```python
from build123d import *

# Parameters (mm, degrees)
SKETCH1_W               = 15
SKETCH1_H               = 7.5
BOSS_EXTRUDE_BASE_DEPTH = 3
SKETCH2_W               = 15
SKETCH2_H               = 2.5
SKETCH2_H_2             = 1.4
BOSS_EXTRUDE2_DEPTH     = 16
CUT_EXTRUDE1_DEPTH      = 26.342651795
SKETCH6_R               = 2.75
CUT_EXTRUDE_HOLE_DEPTH  = 26.342651795
SKETCH7_R               = 5.5
BOSS_EXTRUDE4_DEPTH     = 3
CUT_EXTRUDE4_DEPTH      = 3


with BuildPart() as part:
    # Sketch1 → Boss-Extrude - Base (new body)
    with BuildSketch(Plane(origin=(0, 0, 0), x_dir=(1, 0, 0), z_dir=(0, 1, 0))):
        with Locations((7.5, 3.75)):
            Rectangle(SKETCH1_W, SKETCH1_H)
    extrude(amount=BOSS_EXTRUDE_BASE_DEPTH)

    # Sketch2 → Boss-Extrude2 (add)
    with BuildSketch(Plane(origin=(0, 3, 0), x_dir=(1, 0, 0), z_dir=(0, 1, 0))):
        with Locations((7.5, 6.25)):
            Rectangle(SKETCH2_W, SKETCH2_H)
        with Locations((7.5, 0.7)):
            Rectangle(SKETCH2_W, SKETCH2_H_2)
    extrude(amount=BOSS_EXTRUDE2_DEPTH)

    # Sketch4 → Cut-Extrude1 (cut, through all)
    with BuildSketch(Plane(origin=(0, 0, -7.5), x_dir=(-1, 0, 0), z_dir=(0, 0, -1))):
        with BuildLine():
            Line((0, 3), (3.144969959, 3))
            Line((3.144969959, 3), (3.144969959, 20.655431795))
            Line((3.144969959, 20.655431795), (-18.154935256, 20.655431795))
            Line((-18.154935256, 20.655431795), (-18.154935256, 3))
            Line((-18.154935256, 3), (-15, 3))
            ThreePointArc((-15, 3), (-14.902566102, 3.529038543), (-14.623050239, 3.988653628))
            ThreePointArc((-14.623050239, 3.988653628), (-13.75, 5.91762732), (-14.133249581, 8))
            ThreePointArc((-14.133249581, 8), (-7.5, 19), (-0.866750419, 8))
            ThreePointArc((-0.866750419, 8), (-1.25, 5.91762732), (-0.376949761, 3.988653628))
            ThreePointArc((-0.376949761, 3.988653628), (-0.097433898, 3.529038543), (0, 3))
        make_face()
    extrude(amount=-CUT_EXTRUDE1_DEPTH, mode=Mode.SUBTRACT)

    # Sketch6 → Cut-Extrude - Hole (cut, through all)
    with BuildSketch(Plane(origin=(0, 0, -7.5), x_dir=(-1, 0, 0), z_dir=(0, 0, -1))):
        with Locations((-7.5, 11.5)):
            Circle(SKETCH6_R)
    extrude(amount=-CUT_EXTRUDE_HOLE_DEPTH, mode=Mode.SUBTRACT)

    # Mirror1: part across plane


with BuildPart() as part_1:
    add(part.part)
    add(part.part.mirror(Plane(origin=(0, 3, 0), x_dir=(1, 0, 0), z_dir=(0, 0, -1))))

    # Sketch7 → Boss-Extrude4 (add)
    with BuildSketch(Plane(origin=(0, 0, -7.5), x_dir=(-1, 0, 0), z_dir=(0, 0, -1))):
        with Locations((-7.5, 11.5)):
            Circle(SKETCH7_R)
    extrude(amount=BOSS_EXTRUDE4_DEPTH)

    # Sketch8 → Cut-Extrude4 (cut)
    with BuildSketch(Plane(origin=(0, 0, -10.5), x_dir=(-1, 0, 0), z_dir=(0, 0, -1))):
        Polygon((-3.5, 9.190598923), (-3.5, 13.809401077), (-7.5, 16.118802154), (-11.5, 13.809401077), (-11.5, 9.190598923), (-7.5, 6.881197846), align=None)
    extrude(amount=-CUT_EXTRUDE4_DEPTH, mode=Mode.SUBTRACT)


solid = part_1.part
```
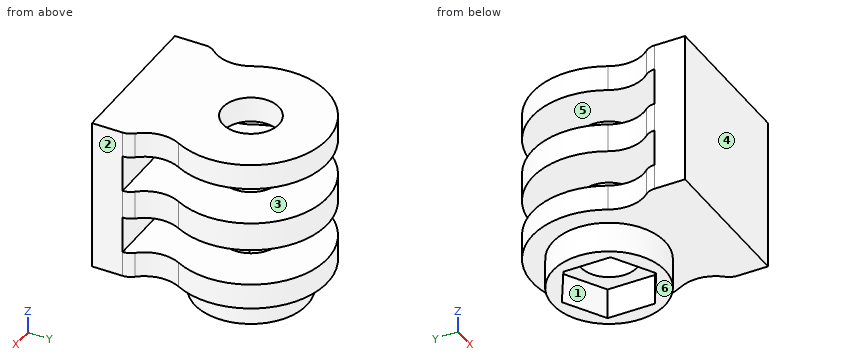
Geometry: final body of the model. Coordinates: model frame, mm. Face numbers are marked on the shaded views. A direction names the side the tool comes from. Round coordinates to 2 decimals unless told otherwise and drop trailing zeros. Order: outer loops, then holes, each group sorted by start corner. A loop starts at its lowest first (then second) coordinate and runs counter-clockwise, first axis right, second up. Notation, with made-up numbers: (7.25, 43.5) -> (50.25, 43.5) arc R24 cw to (50.25, 69.5) -> close; hole circle Ø11 at (20, 76). An arc over 180 degrees is marked (long way). Use one line per item in the form item = value. Start each with the question number.
1. Line query: probe 1 along Z at (x, y) = (13.25, 14); probe 2 along Y at (x, z) = (7.5, -6.95); probe 3 along Z at (x, y) = (10.5, 7). Output: solid intervals per line, ascending.
2. Cut plane D-D (z = -4.5). Return the cut outline in (x, y).
3. Pin query (flat end, axial travel): pin 1 Ø3 at (x, z) = (9.5, 2.5) entering from +Y; pin 2 Ø7 at (x, y) = (7.5, 11.5) entering from -Z; pin 3 Ø1.5 at (y, z) = (10.5, -9) entering from +X. Return the tip coordinate at first contact, or that it passes through.
4. Draft query along Z for the marked faces 4, 5 and 6. Return one class per face: pulls with the +Z half, pulls with the -Z half, needs draft (parallel to the pull), parting line crosses it, or undercut.
5. Cut plane A-A (y = 11.5). Count the separate pieces of the cut face and the enclosed holes in it, then the cut area to 3 significant figures.
6. Reachability of the marked faces 1, 2 and 3 from +Z, -Z, +X, -X, +Y, -Y: full face, straight path, thin tool, end or side. Return the list, or none.
7. Cut plane C-C (y = 17.25). Return the cut outline in (x, z).
Solution:
q1.probe_1 = -7.5 to -5, -1.4 to 1.4, 5 to 7.5
q1.probe_2 = 0 to 8.75, 14.25 to 19
q1.probe_3 = -10.5 to -5, -1.4 to 1.4, 5 to 7.5
q2.outline = (0, 0) -> (15, 0) -> (15, 3) -> (0, 3) -> close
q3.pin_1 = 18.94
q3.pin_2 = -7.5
q3.pin_3 = 12.99
q4.face_4 = needs draft
q4.face_5 = undercut
q4.face_6 = pulls with the -Z half
q5.separate_pieces = 6
q5.enclosed_holes = 0
q5.area = 83.1 mm^2
q6.face_1 = -Z
q6.face_2 = +Z, -Z, +X, +Y, -Y
q6.face_3 = +X, -X, +Y
q7.outline = (2.68, -7.5) -> (12.32, -7.5) -> (12.32, -5) -> (2.68, -5) -> close; (2.68, -1.4) -> (12.32, -1.4) -> (12.32, 1.4) -> (2.68, 1.4) -> close; (2.68, 5) -> (12.32, 5) -> (12.32, 7.5) -> (2.68, 7.5) -> close
